```python
from build123d import *

# Parameters (mm, degrees)
SKETCH1_R           = 15
BOSS_EXTRUDE1_DEPTH = 15
SKETCH2_R           = 10.48
CUT_EXTRUDE1_DEPTH  = 4
CUT_EXTRUDE2_DEPTH  = 5


with BuildPart() as part:
    # Sketch1 → Boss-Extrude1 (new body)
    with BuildSketch(Plane(origin=(0, 0, 0), x_dir=(1, 0, 0), z_dir=(0, 1, 0))):
        with Locations(Location((0, 0, 0), (0, 0, 270))):
            Circle(SKETCH1_R)
    extrude(amount=BOSS_EXTRUDE1_DEPTH)

    # Sketch2 → Cut-Extrude1 (cut)
    with BuildSketch(Plane.XZ):
        with Locations(Location((0, 0, 0), (0, 0, 270))):
            Circle(SKETCH2_R)
    extrude(amount=-CUT_EXTRUDE1_DEPTH, mode=Mode.SUBTRACT)

    # Sketch7 → Cut-Extrude2 (cut)
    with BuildSketch(Plane(origin=(0, 15, 0), x_dir=(1, 0, 0), z_dir=(0, 1, 0))):
        Polygon((0, 5.132643893), (-4.445, 2.566321947), (-4.445, -2.566321947), (0, -5.132643893), (4.445, -2.566321947), (4.445, 2.566321947), align=None)
    extrude(amount=-CUT_EXTRUDE2_DEPTH, mode=Mode.SUBTRACT)


solid = part.part
```
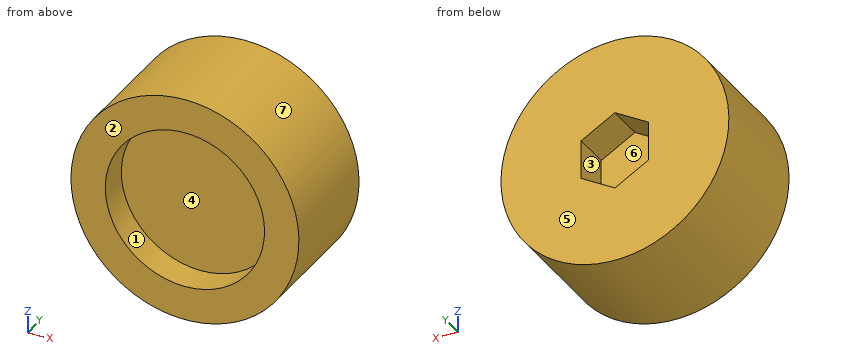
Geometry check sheet. Reference: the model listing, model coordinates, mm. Face numbers are marked on the shaded views. A direction names the side the tool comes from. Round coordinates to 2 decimals unless told otherwise and drop trailing zeros. Loops run counter-clockwise (first coordinate to the right, second up) from the corner with the lowest first, then second, coordinate; pieces in that order, holes last. Notation, with made-up numbers: (-37.5, -5) -> (-17.5, -5) arc R8 cw to (-17.5, 2) -> close; hole circle Ø6 at (78, -33.75). An arc over 180 degrees is marked (long way). Use a Markdown table: item, result.
(1) Sectioned sample at C-C (x = 7.75). Enter the section's corners in (y, z), then the cut area to 3 significant figures.
Calculated:
| item | result |
|---|---|
| outline | (0, -12.84) -> (15, -12.84) -> (15, 12.84) -> (0, 12.84) -> (0, 7.05) -> (4, 7.05) -> (4, -7.05) -> (0, -7.05) -> close |
| area | 329 mm² |
(2) Sectioned sample at A-A (y = 12). Enter the section's corners in (x, z) (3 decimals), then the cut area to 3 significant figures.
Calculated:
| item | result |
|---|---|
| outline | circle Ø30 at (0, 0); hole (-4.445, -2.566) -> (0, -5.133) -> (4.445, -2.566) -> (4.445, 2.566) -> (0, 5.133) -> (-4.445, 2.566) -> close |
| area | 638 mm² |
(3) Sectioned sample at D-D (y = 5.75). Enter the section's corners in (x, z).
Calculated:
| item | result |
|---|---|
| outline | circle Ø30 at (0, 0) |
(4) Mould release check, pull along Z, two halves, no side actions. Record for the marked faces 4, 5, 6 and 7: released by +Z, released by -Z, zero draft, split by the parting line, or undercut.
Calculated:
| item | result |
|---|---|
| face 4 | undercut |
| face 5 | zero draft |
| face 6 | undercut |
| face 7 | split by the parting line |
(5) Go/stop test with flat-tipped pins: P1, Ø8, axis at y = 5, z = -11.5, coming from the +X side; P2, Ø10.5, axis at x = 4.5, z = 0.5, coming from the -Y side; P3, Ø1, axis at x = 3.5, y = 3.5, coming from the -Z side. Record where each tip stops, or that it passes through.
Calculated:
| item | result |
|---|---|
| P1 | x = 12.99 |
| P2 | y = 4 |
| P3 | z = -14.7 |
(6) Set-up check for the marked faces 1, 2 and 3: record each of +Z, -Z, +X, -X, +Y, -Y from which the full face is reachable in a straight line by a thin tool's end or side.
Calculated:
| item | result |
|---|---|
| face 1 | -Y |
| face 2 | +Z, -Z, +X, -X, -Y |
| face 3 | +Y |
(7) Sectioned sample at B-B (z = 0). Enter the section's corners in (x, y) (3 decimals), then the cut area to 3 significant figures.
Calculated:
| item | result |
|---|---|
| outline | (-15, 0) -> (-10.48, 0) -> (-10.48, 4) -> (10.48, 4) -> (10.48, 0) -> (15, 0) -> (15, 15) -> (4.445, 15) -> (4.445, 10) -> (-4.445, 10) -> (-4.445, 15) -> (-15, 15) -> close |
| area | 322 mm² |
(8) Scan lines: probe 1 along X at (y, z) = (2.1, 0); probe 2 along Y at (x, z) = (8, -1.5); probe 3 along Z at (x, y) = (-4, 1.5). Record each from-to range of solid material in increasing order.
Calculated:
| item | result |
|---|---|
| probe 1 | -15 to -10.48, 10.48 to 15 |
| probe 2 | 4 to 15 |
| probe 3 | -14.46 to -9.69, 9.69 to 14.46 |
